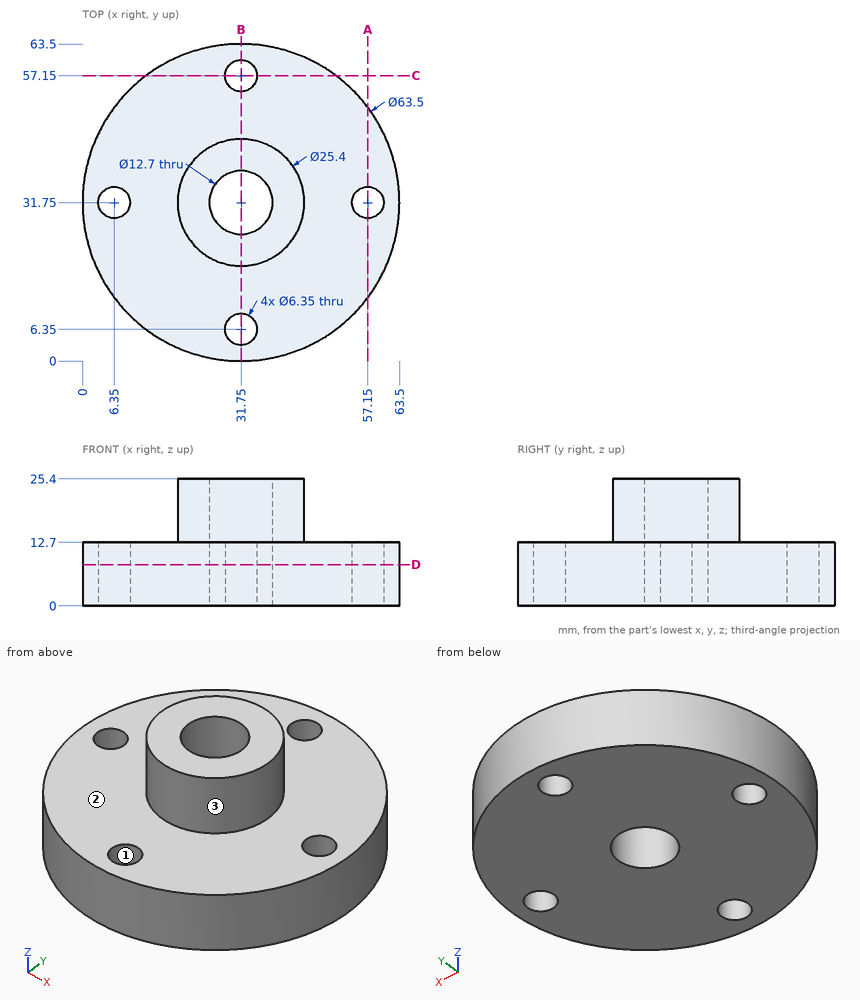
Job drawing, mm, ordinate dimensions from the low corner. One solid piece. Give positions to 0.01 mm unless a question says otherwise; leave off trailing zeros. Order: outer loops, then holes, each group sorted by start corner. A loop starts at its lowest first (then second) coordinate and runs counter-clockwise, first axis right, second up. Notation, with made-up numbers: (13, -29) -> (71, -29) arc R12 cw to (71, -20) -> close; hole circle Ø3 at (31, 1). An arc over 180 degrees is marked (long way). Return JSON: item names as keys, results as strings.
Q1. Drill centre lines: line 1 (Y direction, x = 31.75, z = 5) (3 decimals); line 2 (Z direction, x = 36, y = 44.5); line 3 (X direction, y = 27, z = 18.75). Where is each one in solid material? Low to high.
Working result:
{"line 1": "0 to 3.175, 9.525 to 25.4, 38.1 to 53.975, 60.325 to 63.5", "line 2": "0 to 12.7", "line 3": "19.97 to 27.54, 35.96 to 43.53"}
Q2. Saw through at D-D (z = 8.25). Write the cut outline in (x, y) (3 decimals).
Working result:
{"outline": "circle Ø63.5 at (31.75, 31.75); hole circle Ø6.35 at (6.35, 31.75); hole circle Ø12.7 at (31.75, 31.75); hole circle Ø6.35 at (31.75, 6.35); hole circle Ø6.35 at (31.75, 57.15); hole circle Ø6.35 at (57.15, 31.75)"}
Q3. Saw through at B-B (x = 31.75). Write the cut outline in (y, z) (3 decimals).
Working result:
{"outline": "(0, 0) -> (3.175, 0) -> (3.175, 12.7) -> (0, 12.7) -> close; (9.525, 0) -> (25.4, 0) -> (25.4, 25.4) -> (19.05, 25.4) -> (19.05, 12.7) -> (9.525, 12.7) -> close; (38.1, 0) -> (53.975, 0) -> (53.975, 12.7) -> (44.45, 12.7) -> (44.45, 25.4) -> (38.1, 25.4) -> close; (60.325, 0) -> (63.5, 0) -> (63.5, 12.7) -> (60.325, 12.7) -> close"}
Q4. Saw through at A-A (x = 57.15). Write the cut outline in (y, z) (3 decimals), then the cut area to 3 significant figures.
Working result:
{"outline": "(12.7, 0) -> (28.575, 0) -> (28.575, 12.7) -> (12.7, 12.7) -> close; (34.925, 0) -> (50.8, 0) -> (50.8, 12.7) -> (34.925, 12.7) -> close", "area": "403 mm²"}
Q5. Flat gauge pins, fed straight in: pin 1 (10 mm diameter, centred on x = 6.5, z = 19.5, fed in from -Y); pin 2 (6 mm diameter, centred on y = 21.5, z = 14.5, fed in from -X); pin 3 (12 mm diameter, centred on y = 43.5, z = 3.5, fed in from -X) (3 decimals); pin 4 (20.5 mm diameter, centred on x = 31.75, y = 31.75, fed in from +Z). Where does each tip first touch, or does it go through?
Working result:
{"pin 1": "through", "pin 2": "x = 0.99", "pin 3": "x = 0.525", "pin 4": "z = 25.4"}
Q6. Mould opens along Y. For the marked faces 1, 2 and 3 say: pulls with the +Y half, pulls with the -Y half, needs draft (parallel to the pull), parting line crosses it, or undercut.
Working result:
{"face 1": "undercut", "face 2": "needs draft", "face 3": "parting line crosses it"}
